```python
from build123d import *

# Parameters (mm, degrees)
BOSS_EXTRUDE1_DEPTH  = 8.6
CHAMFER1_SIZE        = 1.414
CHAMFER1_EDGE_2_SIZE = 1.414
CHAMFER1_EDGE_3_SIZE = 1.414
CHAMFER1_EDGE_4_SIZE = 1.414
CHAMFER1_EDGE_5_SIZE = 1.414
CHAMFER1_EDGE_6_SIZE = 1.414
FILLET1_R            = 0.25
SKETCH6_R            = 1.5
CUT_EXTRUDE1_DEPTH   = 28
BOSS_EXTRUDE2_DEPTH  = 2.1
SKETCH9_R            = 2.75
CUT_EXTRUDE2_DEPTH   = 4.2
CHAMFER3_SIZE        = 0.75


with BuildPart() as part:
    # Sketch1 → Revolve1 (revolve)
    with BuildSketch(Plane.XY, mode=Mode.PRIVATE) as revolve1_sk:
        Polygon((0, 0), (6, 0), (6, 5.75), (4.875, 5.75), (4.875, 6.5), (7.75, 8), (7.75, 44.5), (8.7, 44.5), (8.7, 45.5), (0, 45.5), align=None)
    revolve(revolve1_sk.sketch.rotate(Axis((0, 45.5, 0), (0, -1, 0)), 180), axis=Axis((0, 45.5, 0), (0, -1, 0)))

    # Sketch3 → Boss-Extrude1 (add)
    with BuildSketch(Plane(origin=(0, 45.5, 0), x_dir=(1, 0, 0), z_dir=(0, 1, 0))):
        Polygon((0, 9.814954576), (-8.5, 4.907477288), (-8.5, -4.907477288), (0, -9.814954576), (8.5, -4.907477288), (8.5, 4.907477288), align=None)
    extrude(amount=BOSS_EXTRUDE1_DEPTH)

    # Chamfer1
    chamfer1_edges = [part.edges().sort_by_distance(p)[0] for p in [
        (8.5, 49.8, -4.907477288),
    ]]
    chamfer(chamfer1_edges, length=CHAMFER1_SIZE)

    # Chamfer1 edge 2
    chamfer1_edge_2_edges = [part.edges().sort_by_distance(p)[0] for p in [
        (0, 49.8, -9.814954576),
    ]]
    chamfer(chamfer1_edge_2_edges, length=CHAMFER1_EDGE_2_SIZE)

    # Chamfer1 edge 3
    chamfer1_edge_3_edges = [part.edges().sort_by_distance(p)[0] for p in [
        (-8.5, 49.8, -4.907477288),
    ]]
    chamfer(chamfer1_edge_3_edges, length=CHAMFER1_EDGE_3_SIZE)

    # Chamfer1 edge 4
    chamfer1_edge_4_edges = [part.edges().sort_by_distance(p)[0] for p in [
        (-8.5, 49.8, 4.907477288),
    ]]
    chamfer(chamfer1_edge_4_edges, length=CHAMFER1_EDGE_4_SIZE)

    # Chamfer1 edge 5
    chamfer1_edge_5_edges = [part.edges().sort_by_distance(p)[0] for p in [
        (0, 49.8, 9.814954576),
    ]]
    chamfer(chamfer1_edge_5_edges, length=CHAMFER1_EDGE_5_SIZE)

    # Chamfer1 edge 6
    chamfer1_edge_6_edges = [part.edges().sort_by_distance(p)[0] for p in [
        (8.5, 49.8, 4.907477288),
    ]]
    chamfer(chamfer1_edge_6_edges, length=CHAMFER1_EDGE_6_SIZE)

    # Sketch5 → Revolve2 (revolve)
    with BuildSketch(Plane.XY, mode=Mode.PRIVATE) as revolve2_sk:
        Polygon((7.75, 34.901965379), (10.5, 34.901965379), (10.5, 32.901965379), (8.7, 32.901965379), (8.7, 29.901965379), (7.75, 29.901965379), align=None)
    revolve(revolve2_sk.sketch.rotate(Axis((0, 0, 0), (0, 1, 0)), 180), axis=Axis((0, 0, 0), (0, 1, 0)))

    # Fillet1
    fillet1_edges = [part.edges().sort_by_distance(p)[0] for p in [
        (10.5, 34.901965379, 0),
        (10.5, 32.901965379, 0),
        (8.7, 29.901965379, 0),
    ]]
    fillet(fillet1_edges, radius=FILLET1_R)

    # Sketch6 → Cut-Extrude1 (cut)
    with BuildSketch(Plane.XZ):
        Circle(SKETCH6_R)
    extrude(amount=-CUT_EXTRUDE1_DEPTH, mode=Mode.SUBTRACT)

    # Sketch7 → Boss-Extrude2 (add, symmetric)
    with BuildSketch(Plane.XY):
        with BuildLine():
            Line((4.5, 60.35), (4.5, 54.1))
            Line((4.5, 54.1), (-4.5, 54.1))
            Line((-4.5, 54.1), (-4.5, 60.35))
            ThreePointArc((-4.5, 60.35), (0, 64.85), (4.5, 60.35))
        make_face()
    extrude(amount=BOSS_EXTRUDE2_DEPTH, both=True)

    # Sketch8 → Cut-Revolve1 (revolve, cut)
    with BuildSketch(Plane.XY):
        with BuildLine():
            Line((0, 63.25), (0, 57.45))
            ThreePointArc((0, 57.45), (2.9, 60.35), (0, 63.25))
        make_face()
    revolve(axis=Axis((0, 54.1, 0), (0, 1, 0)), mode=Mode.SUBTRACT)

    # Sketch9 → Cut-Extrude2 (cut)
    with BuildSketch(Plane.XY.offset(2.1)):
        with Locations((0, 60.35)):
            Circle(SKETCH9_R)
    extrude(amount=-CUT_EXTRUDE2_DEPTH, mode=Mode.SUBTRACT)

    # Sketch10 → Cut-Revolve2 (revolve, cut)
    with BuildSketch(Plane.XY, mode=Mode.PRIVATE) as cut_revolve2_sk:
        Polygon((7, 54.1), (8.5, 52.7), (10.124681139, 51.183630937), (10.124681139, 53.919402207), (7, 56.83577127), align=None)
    revolve(cut_revolve2_sk.sketch.rotate(Axis((0, 0, 0), (0, 1, 0)), 90), axis=Axis((0, 0, 0), (0, 1, 0)), mode=Mode.SUBTRACT)

    # Chamfer3
    chamfer3_edges = [part.edges().sort_by_distance(p)[0] for p in [
        (6, 0, 0),
    ]]
    chamfer(chamfer3_edges, length=CHAMFER3_SIZE)


solid = part.part
```
Can you work these out from the model? Positions are in its coordinate system, mm. A direction names the side the tool comes from. Coordinates: 2 decimals unless noted, no trailing zeros. Loops run counter-clockwise (first coordinate to the right, second up) from the corner with the lowest first, then second, coordinate; pieces in that order, holes last. Notation, with made-up numbers: (48.25, 79.25) - (90.25, 79.25) arc R20 ccw to (90.25, 89.25) - close; hole circle Ø6 at (-2.5, -17). An arc over 180 degrees is marked (long way). Answer as CSV lines item,"result". Start each with the question number.
1) Which directions (+Z, -Z, +X, -X, +Y, -Y) give clear straight access to the entire face, cutting with the end or side of a thin tool? Please do faces 5 (the flat face through (0, 57, 2.1)), 6 (the flat face through (-8, 44.5, 1)), 7 (the flat face through (-4.29, 49.05, 7.34)).
2) Suppose I cut it at B-B (y = 15). Please give me the cut outline in (x, z).
3) Suppose I cut it at C-C (y = 40.5). Please give me the cut outline in (x, z), plus the area to 3 significant figures.
4) Thinking about a two-plate mould opening in Y: for faces 1 (the flat face through (-7.896, 48.77, -4.539)), 2 (the cylindrical face through (-0.1, 64.85, 0.03)), 3 (the cylindrical face through (-0.596, 57.665, -1.502)), 4 (the cylindrical face through (0.635, 6.13, -4.834)), which applies, pulls with the +Y half, pulls with the -Y half, needs draft (parallel to the pull), parting line crosses it, or undercut?
5) I need wall thicknesses on line 1 (Z direction, x = 0, y = 11.75); line 2 (Y direction, x = 0, z = -1.2); line 3 (X direction, y = 60.35, z = 1.65). Which ranges of each line are inside material? Lowest first, please. Write a range as from..to.
6) For pin 1 (5 mm diameter, centred on x = -4.5, y = 38, fed in from +Z); pin 2 (10 mm diameter, centred on x = 4.5, z = -1.5, fed in from +Y); pin 3 (1.5 mm diameter, centred on x = 0, y = 18, fed in from +Z); pin 4 (0.6 mm diameter, centred on x = -4, z = -7, fed in from +Y), each with a flat end and sliding along its axis, tell me the tip position at first contact or that it passes through.
7) Suppose I cut it at A-A (y = 31.5). Please give me the cut outline in (x, z).
Check result:
1,face 5,"+Z, +X, -X, +Y"
1,face 6,"none"
1,face 7,"+Z, -X, +Y"
2,outline,"circle Ø15.5 at (0, 0); hole circle Ø3 at (0, 0)"
3,outline,"circle Ø15.5 at (0, 0)"
3,area,"189 mm²"
4,face 1,"needs draft"
4,face 2,"pulls with the +Y half"
4,face 3,"undercut"
4,face 4,"undercut"
5,line 1,"z = -7.75..-1.5, 1.5..7.75"
5,line 2,"y = 28..57.6, 63.1..64.85"
5,line 3,"x = -4.5..-2.75, 2.75..4.5"
6,pin 1,"stops at z = 7.49"
6,pin 2,"stops at y = 64.85"
6,pin 3,"stops at z = 7.75"
6,pin 4,"stops at y = 53.39"
7,outline,"circle Ø17.4 at (0, 0)"
